The figure shows three views and two pictorial views of one solid part (mm, origin at its lowest corner). Answer the questions. A direction names the side the tool comes from. Coordinates: 2 decimals unless noted, no trailing zeros. Loops run counter-clockwise (first coordinate to the right, second up) from the corner with the lowest first, then second, coordinate; pieces in that order, holes last. Notation, with made-up numbers: (89, 58) - (122, 58) arc R29 ccw to (122, 97) - close; hole circle Ø10 at (-11, 46.25). An arc over 180 degrees is marked (long way). Return JSON: item names as keys, results as strings. Group by question number.
1. Section B-B (z = 98) is taken. Write down the section's boundary in (x, y), and give its area (3 significant figures).
2. Find the intervals of material crossed by line 1 along Z through (x, y) = (50, 63); line 2 along X through (y, z) = (59, 76); line 3 along X through (y, z) = (71, 82), in increasing order.
3. Section D-D (z = 9) is taken. Write down the section's boundary in (x, y), and give its area (3 significant figures).
4. Each of these flat-tipped pins is pushed along its axis until it touches: P1, Ø2, axis at y = 51, z = 86, coming from the +X side; P2, Ø10, axis at y = 45.5, z = 56.5, coming from the +X side; P3, Ø10, axis at x = 32, y = 65, coming from the +Z side; P4, Ø15, axis at x = 62.5, y = 34, coming from the +Z side. Where does it stop, or does it pass through?
5. The mould has two halves that part along X. Classify the marked faces 1, 2 and 3: pulls with the +X half, pulls with the -X half, needs draft (parallel to the pull), parting line crosses it, or undercut.
6. Which of the six approach directions +Z, -Z, +X, -X, +Y, -Y give full straight-line access (tool end or side, diameter ignored) to the marked faces 4, 5 and 6?
7. Section C-C (x = 47) is taken. Write down the section's boundary in (y, z), and give its area (3 significant figures).
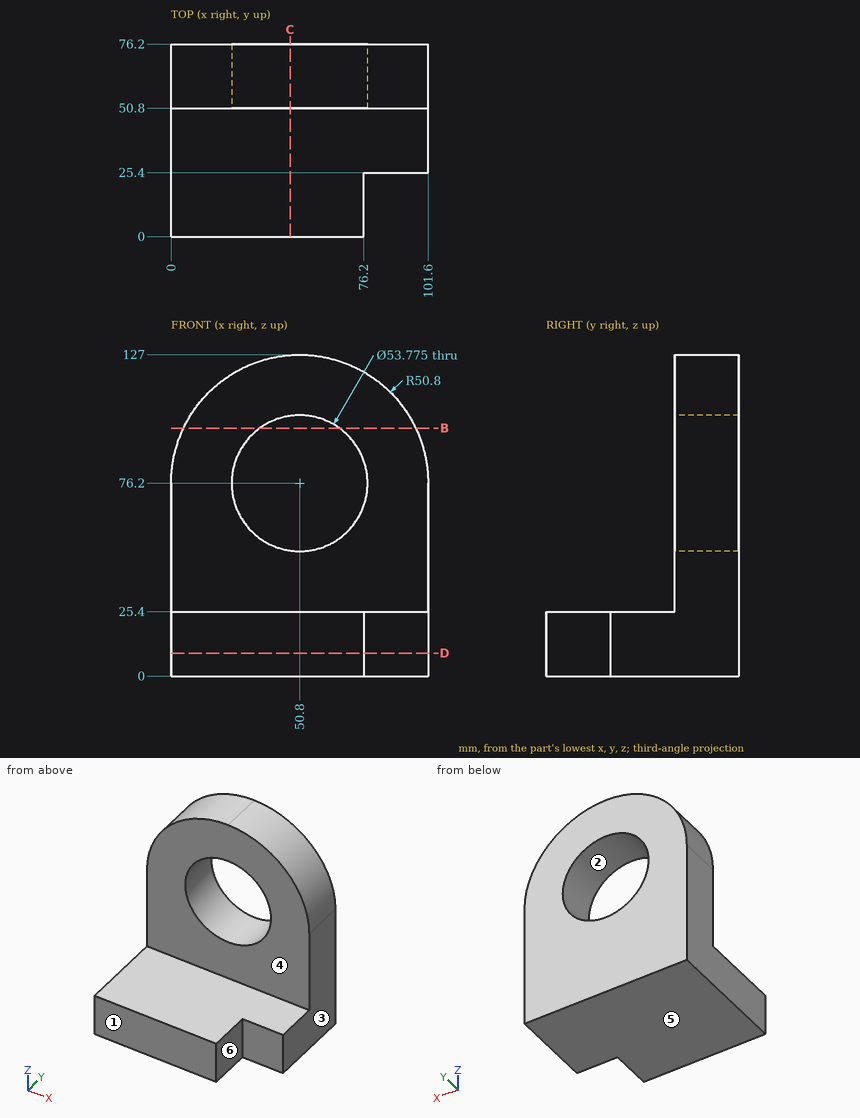
The answers:
{
 "1": {"outline": "(4.92, 50.8) - (35.06, 50.8) - (35.06, 76.2) - (4.92, 76.2) - close; (66.54, 50.8) - (96.68, 50.8) - (96.68, 76.2) - (66.54, 76.2) - close", "area": "1,530 mm2"},
 "2": {"line 1": "z = 0 to 49.32, 103.08 to 126.99", "line 2": "x = 0 to 23.91, 77.69 to 101.6", "line 3": "x = 0.33 to 24.55, 77.05 to 101.27"},
 "3": {"outline": "(0, 0) - (76.2, 0) - (76.2, 25.4) - (101.6, 25.4) - (101.6, 76.2) - (0, 76.2) - close", "area": "7,100 mm2"},
 "4": {"P1": "stops at x = 100.83", "P2": "passes through", "P3": "stops at z = 125.09", "P4": "stops at z = 25.4"},
 "5": {"face 1": "needs draft", "face 2": "undercut", "face 3": "pulls with the +X half"},
 "6": {"face 4": "+Z, +X, -X, -Y", "face 5": "-Z, +X, -X, +Y, -Y", "face 6": "+Z, -Z, +X, -Y"},
 "7": {"outline": "(0, 0) - (76.2, 0) - (76.2, 49.58) - (50.8, 49.58) - (50.8, 25.4) - (0, 25.4) - close; (50.8, 102.82) - (76.2, 102.82) - (76.2, 126.86) - (50.8, 126.86) - close", "area": "3,160 mm2"}
}
